from build123d import *

# Parameters (mm, degrees)
SKIZZE1_W                       = 243
SKIZZE1_H                       = 151
SKIZZE1_W_2                     = 203
SKIZZE1_H_2                     = 125
AUFSATZ_LINEAR_AUSTRAGEN1_DEPTH = 2
SKIZZE2_W                       = 243
SKIZZE2_H                       = 151
SKIZZE2_W_2                     = 239
SKIZZE2_H_2                     = 147
AUFSATZ_LINEAR_AUSTRAGEN2_DEPTH = 14.5
SKIZZE3_R                       = 1.75
SCHNITT_LINEAR_AUSTRAGEN1_DEPTH = 287.461603012
VERRUNDUNG1_R                   = 2
VERRUNDUNG2_R                   = 4
VERRUNDUNG3_R                   = 1


with BuildPart() as part:
    # Skizze1 → Aufsatz-Linear austragen1 (new body)
    with BuildSketch(Plane(origin=(0, 0, 0), x_dir=(1, 0, 0), z_dir=(0, 1, 0))):
        with Locations((121.5, 75.5)):
            Rectangle(SKIZZE1_W, SKIZZE1_H)
        with Locations((121.5, 76.5)):
            Rectangle(SKIZZE1_W_2, SKIZZE1_H_2, mode=Mode.SUBTRACT)
    extrude(amount=AUFSATZ_LINEAR_AUSTRAGEN1_DEPTH)

    # Skizze2 → Aufsatz-Linear austragen2 (add)
    with BuildSketch(Plane(origin=(0, 2, 0), x_dir=(1, 0, 0), z_dir=(0, 1, 0))):
        with Locations((121.5, 75.5)):
            Rectangle(SKIZZE2_W, SKIZZE2_H)
        with Locations((121.5, 75.5)):
            Rectangle(SKIZZE2_W_2, SKIZZE2_H_2, mode=Mode.SUBTRACT)
    extrude(amount=AUFSATZ_LINEAR_AUSTRAGEN2_DEPTH)

    # Skizze3 → Schnitt-Linear austragen1 (cut, through all)
    with BuildSketch(Plane(origin=(0, 2, 0), x_dir=(1, 0, 0), z_dir=(0, 1, 0))):
        with Locations(Location((15.23, 142, 0), (0, 0, 270))):
            Circle(SKIZZE3_R)
        with Locations(Location((233.33, 142, 0), (0, 0, 270))):
            Circle(SKIZZE3_R)
        with Locations(Location((15.23, 9, 0), (0, 0, 270))):
            Circle(SKIZZE3_R)
        with Locations(Location((233.33, 9, 0), (0, 0, 270))):
            Circle(SKIZZE3_R)
    extrude(amount=-SCHNITT_LINEAR_AUSTRAGEN1_DEPTH, mode=Mode.SUBTRACT)

    # Verrundung1
    verrundung1_edges = [part.edges().sort_by_distance(p)[0] for p in [
        (2, 9.25, -2),
        (241, 9.25, -2),
        (241, 9.25, -149),
        (2, 9.25, -149),
    ]]
    fillet(verrundung1_edges, radius=VERRUNDUNG1_R)

    # Verrundung2
    verrundung2_edges = [part.edges().sort_by_distance(p)[0] for p in [
        (0, 8.25, -151),
        (243, 8.25, -151),
        (243, 8.25, 0),
        (0, 8.25, 0),
    ]]
    fillet(verrundung2_edges, radius=VERRUNDUNG2_R)

    # Verrundung3
    verrundung3_edges = [part.edges().sort_by_distance(p)[0] for p in [
        (121.5, 16.5, -151),
        (121.5, 16.5, 0),
        (243, 16.5, -75.5),
        (1.171572875, 16.5, -1.171572875),
        (241.828427125, 16.5, -1.171572875),
        (241.828427125, 16.5, -149.828427125),
        (1.171572875, 16.5, -149.828427125),
        (0, 16.5, -75.5),
    ]]
    fillet(verrundung3_edges, radius=VERRUNDUNG3_R)


solid = part.part
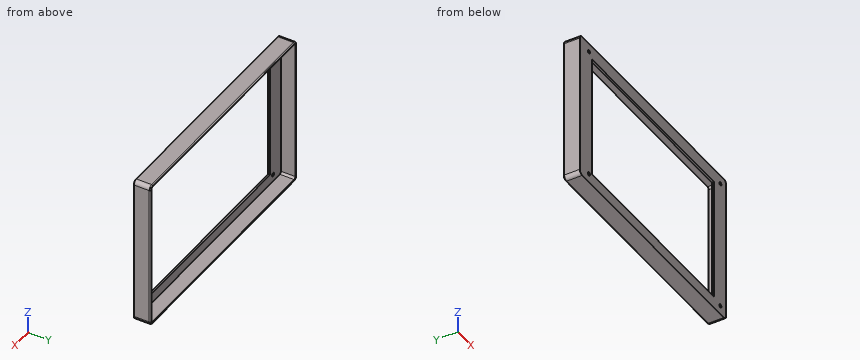
For this review, take the finished solid that the model builds, in its own axes (mm). Coordinates: 2 decimals unless noted, no trailing zeros. Write each loop counter-clockwise with the first axis right and the second up, starting at its lowest first coordinate (ties: lowest second). Pieces come first, ordered by that corner, then holes. Notation, with made-up numbers: (87, 48) -> (94, 48) arc R21 ccw to (94, 80) -> close; hole circle Ø5 at (-30, 31). An arc over 180 degrees is marked (long way). Write each question's results on one line, items separated by ' | '. Start each with the question number.
1) Consider section B-B (z = -87). Write out the cut boundary in (x, y), plus the area to 3 significant figures.
2) Consider section C-C (y = 9). Write out the cut boundary in (x, z).
3) Consider section A-A (x = 68). Write out the cut boundary in (y, z), plus the area to 3 significant figures.
4) Wall thickness on L1, parallel to X at y = 1.6, z = -142; L2, parallel to Z at x = 233.33, y = 1.4; L3, parallel to X at y = 11.5, z = -109: over which ranges is each line inside the solid? List them lowest first. Write a range as [from, to].
5) Insertion check: pin 1 (3 mm diameter, centred on x = 15.23, z = -142, fed in from +Y). The pin has a flat end and moves straight along its axis. Give the tip position at first contact, or say it passes through.
Geometry says:
1) outline: (0, 0) -> (20, 0) -> (20, 2) -> (2, 2) -> (2, 16.5) -> (1, 16.5) arc R1 ccw to (0, 15.5) -> close; (223, 0) -> (243, 0) -> (243, 15.5) arc R1 ccw to (242, 16.5) -> (241, 16.5) -> (241, 2) -> (223, 2) -> close | area: 138 mm^2
2) outline: (0, -147) arc R4 ccw to (4, -151) -> (239, -151) arc R4 ccw to (243, -147) -> (243, -4) arc R4 ccw to (239, 0) -> (4, 0) arc R4 ccw to (0, -4) -> close; hole (2, -147) arc R2 ccw to (4, -149) -> (239, -149) arc R2 ccw to (241, -147) -> (241, -4) arc R2 ccw to (239, -2) -> (4, -2) arc R2 ccw to (2, -4) -> close
3) outline: (0, -151) -> (15.5, -151) arc R1 ccw to (16.5, -150) -> (16.5, -149) -> (2, -149) -> (2, -139) -> (0, -139) -> close; (0, -14) -> (2, -14) -> (2, -2) -> (16.5, -2) -> (16.5, -1) arc R1 ccw to (15.5, 0) -> (0, 0) -> close | area: 110 mm^2
4) L1: [0, 13.48], [16.98, 231.58], [235.08, 243] | L2: [-151, -143.75], [-140.25, -10.75], [-7.25, 0] | L3: [0, 2], [241, 243]
5) pin 1: through
